Design review of the part built by this model. Coordinates are the model's own, in mm. Face numbers are marked on the shaded views. A direction names the side the tool comes from. Give positions to 0.01 mm unless a question says otherwise; leave off trailing zeros. Loops run counter-clockwise (first coordinate to the right, second up) from the corner with the lowest first, then second, coordinate; pieces in that order, holes last. Notation, with made-up numbers: (83, -10) -> (129, -10) arc R8 ccw to (129, -4) -> close; hole circle Ø9 at (36.5, 20). An arc over 180 degrees is marked (long way). Use a Markdown table: item, result. Add a question column.
1. To check wall thickness, follow line 1 (Y direction, x = 0, z = 3.2); line 2 (Y direction, x = 0, z = 0.35); line 3 (Y direction, x = 0, z = 0.45). State the ranges of each line that lie inside material, in increasing order.
2. For pin 1 Ø6.5 at (x, y) = (-1.5, 2) entering from +Z; pin 2 Ø12 at (x, y) = (7, -7.5) entering from -Z; pin 3 Ø1.5 at (y, z) = (-2.5, 4.5) entering from -X, all flat-tipped, find the tip position at first contact; note any pin that passes through.
3. For the marked faces 1 and 2, list the 3-axis set-ups (+Z, -Z, +X, -X, +Y, -Y) from which the entire face can be reached by the end or side of a thin tool; tool diameter is ignored.
4. Draft analysis for pull direction Y (two halves, no side actions). For the marked faces 3 and 4, state which applies: pulls with the +Y half, pulls with the -Y half, needs draft (parallel to the pull), parting line crosses it, or undercut.
5. Add section C-C (z = 3). State the section outline as (x, y) points.
```python
from build123d import *

# Parameters (mm, degrees)
ESBO_O1_R                = 12
ESBO_O1_R_2              = 7.55
RESSALTO_EXTRUS_O1_DEPTH = 5
ESBO_O2_R                = 11.05
ESBO_O2_R_2              = 9.05
CORTE_EXTRUS_O1_DEPTH    = 0.5
ESBO_O3_R                = 11.05
ESBO_O3_R_2              = 9.05
CORTE_EXTRUS_O2_DEPTH    = 0.5
CHANFRO1_SIZE            = 0.5


with BuildPart() as part:
    # Esboço1 → Ressalto-extrusão1 (new body)
    with BuildSketch(Plane.XY):
        Circle(ESBO_O1_R)
        Circle(ESBO_O1_R_2, mode=Mode.SUBTRACT)
    extrude(amount=RESSALTO_EXTRUS_O1_DEPTH)

    # Esboço2 → Corte-extrusão1 (cut)
    with BuildSketch(Plane.XY.offset(5)):
        Circle(ESBO_O2_R)
        Circle(ESBO_O2_R_2, mode=Mode.SUBTRACT)
    extrude(amount=-CORTE_EXTRUS_O1_DEPTH, mode=Mode.SUBTRACT)

    # Esboço3 → Corte-extrusão2 (cut)
    with BuildSketch(Plane(origin=(0, 0, 0), x_dir=(-1, 0, 0), z_dir=(0, 0, -1))):
        Circle(ESBO_O3_R)
        Circle(ESBO_O3_R_2, mode=Mode.SUBTRACT)
    extrude(amount=-CORTE_EXTRUS_O2_DEPTH, mode=Mode.SUBTRACT)

    # Chanfro1
    chanfro1_edges = [part.edges().sort_by_distance(p)[0] for p in [
        (-12, 0, 0),
        (-12, 0, 5),
        (-7.55, 0, 0),
        (-7.55, 0, 5),
    ]]
    chamfer(chanfro1_edges, length=CHANFRO1_SIZE)


solid = part.part
```
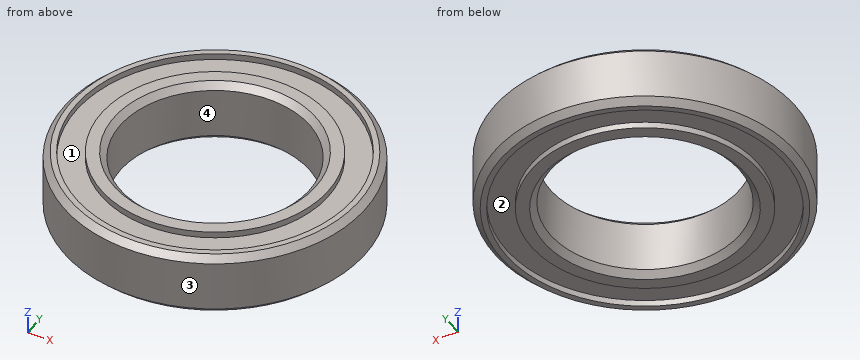
Taken from the geometry:
| question | item | result |
|---|---|---|
| 1 | line 1 | y = -12 to -7.55, 7.55 to 12 |
| 1 | line 2 | y = -11.85 to -11.05, -9.05 to -7.7, 7.7 to 9.05, 11.05 to 11.85 |
| 1 | line 3 | y = -11.95 to -11.05, -9.05 to -7.6, 7.6 to 9.05, 11.05 to 11.95 |
| 2 | pin 1 | passes through |
| 2 | pin 2 | stops at z = 0 |
| 2 | pin 3 | stops at x = -11.87 |
| 3 | face 1 | +Z |
| 3 | face 2 | -Z |
| 4 | face 3 | parting line crosses it |
| 4 | face 4 | undercut |
| 5 | outline | circle Ø24 at (0, 0); hole circle Ø15.1 at (0, 0) |
